from build123d import *

# Parameters (mm, degrees)
F0_W     = 20
F0_H     = 50
F1_DEPTH = 60
F2_R     = 2.5
F3_DEPTH = 20
F4_R     = 5
F5_DEPTH = 80


with BuildPart() as f1:
    # F0 (on Top) → F1 (new body)
    with BuildSketch(Plane.XY):
        Rectangle(F0_W, F0_H)
    extrude(amount=F1_DEPTH)

    # F2 (on face) → F3 (cut)
    with BuildSketch(Plane.XZ.offset(25)):
        with Locations((0, 50)):
            Circle(F2_R)
        with Locations((0, 10)):
            Circle(F2_R)
    extrude(amount=-F3_DEPTH, mode=Mode.SUBTRACT)

    # F4 (on face) → F5 (join)
    with BuildSketch(Plane(origin=(0, 25, 0), x_dir=(-1, 0, 0), z_dir=(0, 1, 0))):
        with Locations((0, 30)):
            Circle(F4_R)
    extrude(amount=F5_DEPTH)


solid = f1.part
For this review, take the finished solid that the model builds, in its own axes (mm). A direction names the side the tool comes from. Coordinates: 2 decimals unless noted, no trailing zeros. Order: outer loops, then holes, each group sorted by start corner. A loop starts at its lowest first (then second) coordinate and runs counter-clockwise, first axis right, second up. Notation, with made-up numbers: (44, 0.5) - (68, 0.5) arc R20 cw to (68, 30.5) - close; hole circle Ø1 at (-11, 85.25). An arc over 180 degrees is marked (long way). Answer as CSV lines item,"result". Start each with the question number.
1) To check wall thickness, follow line 1 along Z through (x, y) = (0, -10); line 2 along Y through (x, z) = (0.5, 47.5); line 3 along Z through (x, y) = (-0.25, 56). State the ranges of each line that lie inside material, in increasing order. Write a range as [from, to].
2) Machinability: for faces 5 (the flat face through (0, -25, 30)), 6 (the flat face through (0, -5, 50)), 7 (the cylindrical face through (1.08, 64.44, 25.12)), which of the approach directions +Z, -Z, +X, -X, +Y, -Y give a long, thin tool a straight path to every point of the face, cutting with its end or side? Answer none if there is none.
3) Add section A-A (z = 10). State the section outline as (x, y) points.
4) Insertion check: P1, Ø6.5, axis at x = 0, z = 50, coming from the +Y side; P2, Ø2.5, axis at x = 1, z = 10.5, coming from the -Y side; P3, Ø10, axis at x = 7, y = 39, coming from the -Z side. Each pin has a flat end and moves straight along its axis. Give the tip position at first contact, or say it passes through.
5) Add section B-B (x = -0.75). State the section outline as (y, z) points.
6) Add section D-D (z = 30). State the section outline as (x, y) points.
7) Add section C-C (y = 73). State the section outline as (x, z) points.
8) Draft analysis for pull direction X (two halves, no side actions). For faces 1 (the flat face through (-10, 0, 30)), 2 (the flat face through (0, 25, 36)), 3 (the flat face through (0, -5, 10)), 4 (the cylindrical face through (-0.54, -15.14, 7.56)), state which applies: +X half, -X half, draft (parallel to the pull), parting line (faces both ways), or undercut.
Result:
1,line 1,"[0, 7.5], [12.5, 47.5], [52.5, 60]"
1,line 2,"[-25, 25]"
1,line 3,"[25.01, 34.99]"
2,face 5,"+Z, -Z, +X, -X, -Y"
2,face 6,"-Y"
2,face 7,"+Y"
3,outline,"(-10, -25) - (-2.5, -25) - (-2.5, -5) - (2.5, -5) - (2.5, -25) - (10, -25) - (10, 25) - (-10, 25) - close"
4,P1,"y = 25"
4,P2,"y = -5"
4,P3,"z = 25.42"
5,outline,"(-25, 0) - (25, 0) - (25, 25.06) - (105, 25.06) - (105, 34.94) - (25, 34.94) - (25, 60) - (-25, 60) - (-25, 52.38) - (-5, 52.38) - (-5, 47.62) - (-25, 47.62) - (-25, 12.38) - (-5, 12.38) - (-5, 7.62) - (-25, 7.62) - close"
6,outline,"(-10, -25) - (10, -25) - (10, 25) - (5, 25) - (5, 105) - (-5, 105) - (-5, 25) - (-10, 25) - close"
7,outline,"circle Ø10 at (0, 30)"
8,face 1,"-X half"
8,face 2,"draft"
8,face 3,"undercut"
8,face 4,"undercut"
